Work out the finished part from the listing and answer in its coordinate system (mm). A direction names the side the tool comes from. Round coordinates to 2 decimals unless told otherwise and drop trailing zeros. Loops run counter-clockwise (first coordinate to the right, second up) from the corner with the lowest first, then second, coordinate; pieces in that order, holes last. Notation, with made-up numbers: (-35.75, 19.25) - (-4.75, 19.25) arc R12 ccw to (-4.75, 37.25) - close; hole circle Ø7 at (-3.5, 5.5). An arc over 180 degrees is marked (long way). Answer as CSV lines item,"result". Start each with the question number.
Q1. Section C-C on y = 30.5 is taken. Write down the section's boundary in (x, z).
Q2. Section B-B on y = 19.5 is taken. Write down the section's boundary in (x, z).
Q3. Section D-D on x = -18 is taken. Write down the section's boundary in (y, z).
Q4. The mould has two halves that part along X. Classify faces 4 (the face through (-50, 25, 1)), 5 (the face through (45, 14, -39)), 6 (the face through (-1, 0, -1)): +X half, -X half, draft (parallel to the pull), parting line (faces both ways), or undercut.
Q5. For faces 1 (the face through (50, 25, -1)), 2 (the face through (-47, 28, 1)), 3 (the face through (-37, 29.123, -38)), determine the directions among +Z, -Z, +X, -X, +Y, -Y from which every point of the face is accessible in a straight line to the end or side of a thin tool.
Q6. Straight lines are drawn through the part: L1, parallel to X at y = 14, z = 23.5; L2, parallel to Z at x = 26, y = 12; L3, parallel to Y at x = 23.5, z = 8.5. For each, find the intervals that lie inside material, in ascending order. Write a range as [from, to].
Q7. Section A-A on x = 43.5 is taken. Write down the section's boundary in (y, z), then the cut area to 3 significant figures.
Autodesk Fusion 360 part; units mm, degrees
sketch "Sketch1" plane through (0, 0, 0) normal (0, 1, 0) x (1, 0, 0)
  line L0 (50, -40) -> (-50, -40)
  line L1 (-50, -40) -> (-50, 40)
  line L2 (-50, 40) -> (50, 40)
  line L3 (50, 40) -> (50, -40)
  line L4 (50, -40) -> (-50, 40) construction
  line L5 (-50, -40) -> (50, 40) construction
  dimension "d1" = 100
  dimension "d2" = 80
extrude "Extrude1" add sketch "Sketch1" along normal blind 50
sketch "Sketch2" plane through (0, 50, 0) normal (0, 1, 0) x (-1, 0, 0)
  line L0 (-50, -40) -> (50, -40)
  line L1 (50, -40) -> (50, 40)
  line L2 (50, 40) -> (-50, 40)
  line L3 (-50, 40) -> (-50, -40)
  line L4 (-47, 37) -> (47, 37)
  line L5 (47, 37) -> (47, -37)
  line L6 (47, -37) -> (-47, -37)
  line L7 (-47, -37) -> (-47, 37)
  line L8 (-47, 37) -> (47, -37) construction
  line L9 (47, 37) -> (-47, -37) construction
  dimension "d5" = 94
  dimension "d6" = 74
  dimension "d15" = 3
  dimension "d16" = 3
extrude "Extrude4" cut sketch "Sketch2" against normal blind 45 contours L4 L5 L6 L7
sketch "Sketch5" plane through (0, 0, -37) normal (0, 0, 1) x (1, 0, 0)
  line L0 (47, 50) -> (-47, 50)
  line L1 (-47, 50) -> (-47, 5)
  line L2 (-47, 5) -> (47, 5)
  line L3 (47, 5) -> (47, 50)
  line L4 (-42.8809, 29.1227) -> (-30.0809, 29.1227)
  line L5 (-30.0809, 29.1227) -> (-30.0809, 10.7227)
  line L6 (-30.0809, 10.7227) -> (-42.8809, 10.7227)
  line L7 (-42.8809, 10.7227) -> (-42.8809, 29.1227)
  dimension "d19" = 12.8
  dimension "d20" = 18.4
extrude "Extrude5" cut sketch "Sketch5" against normal blind 55 contours L4 L5 L6 L7
extrude "Extrude2" cut sketch "Sketch2" against normal blind 45 contours L4 L5 L6 L7
sketch "Sketch3" plane through (0, 0, -40) normal (0, 0, -1) x (-1, 0, 0)
  line L0 (-50, 0) -> (50, 0)
  line L1 (50, 0) -> (50, 50)
  line L2 (50, 50) -> (-50, 50)
  line L3 (-50, 50) -> (-50, 0)
  line L4 (-45, 5) -> (-32.2, 5)
  line L5 (-32.2, 5) -> (-32.2, 23.4)
  line L6 (-32.2, 23.4) -> (-45, 23.4)
  line L7 (-45, 23.4) -> (-45, 5)
  dimension "d11" = 12.8
  dimension "d12" = 18.4
extrude "Extrude3" cut sketch "Sketch3" against normal blind 10 contours L4 L5 L6 L7
Findings:
1,outline,"(-50, -40) - (50, -40) - (50, 40) - (-50, 40) - close; hole (-47, -37) - (47, -37) - (47, 37) - (-47, 37) - close"
2,outline,"(-50, -40) - (-42.88, -40) - (-42.88, -37) - (-47, -37) - (-47, 37) - (47, 37) - (47, -37) - (45, -37) - (45, -40) - (50, -40) - (50, 40) - (-50, 40) - close; (-30.08, -40) - (32.2, -40) - (32.2, -37) - (-30.08, -37) - close"
3,outline,"(0, -40) - (50, -40) - (50, -37) - (5, -37) - (5, 37) - (50, 37) - (50, 40) - (0, 40) - close"
4,face 4,"-X half"
4,face 5,"undercut"
4,face 6,"draft"
5,face 1,"+Z, -Z, +X, +Y, -Y"
5,face 2,"+Y"
5,face 3,"-Z"
6,L1,"x = [-50, -47], [47, 50]"
6,L2,"z = [-40, -37], [37, 40]"
6,L3,"y = [0, 5]"
7,outline,"(0, -40) - (5, -40) - (5, 37) - (50, 37) - (50, 40) - (0, 40) - close; (23.4, -40) - (50, -40) - (50, -37) - (23.4, -37) - close"
7,area,"615 mm^2"
